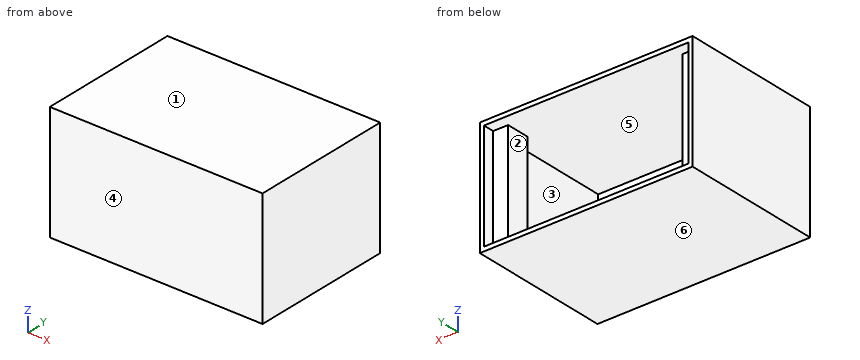
from build123d import *

# Parameters (mm, degrees)
SKETCH1_W           = 456
SKETCH1_H           = 249
SKETCH1_W_2         = 438
SKETCH1_H_2         = 231
BOSS_EXTRUDE1_DEPTH = 9
SKETCH1_3_W         = 456
SKETCH1_3_H         = 249
SKETCH1_3_W_2       = 438
SKETCH1_3_H_2       = 231
BOSS_EXTRUDE2_DEPTH = 298
SKETCH3_W           = 231
SKETCH3_H           = 50
BOSS_EXTRUDE3_DEPTH = 32


with BuildPart() as part:
    # Sketch1 → Boss-Extrude1 (new body)
    with BuildSketch(Plane(origin=(0, 0, 0), x_dir=(1, 0, 0), z_dir=(0, 1, 0))):
        Rectangle(SKETCH1_W, SKETCH1_H)
        Rectangle(SKETCH1_W_2, SKETCH1_H_2, mode=Mode.SUBTRACT)
        Rectangle(SKETCH1_W_2, SKETCH1_H_2)
    extrude(amount=-BOSS_EXTRUDE1_DEPTH)

    # Sketch1<3> → Boss-Extrude2 (add)
    with BuildSketch(Plane(origin=(0, 0, 0), x_dir=(1, 0, 0), z_dir=(0, 1, 0))):
        Rectangle(SKETCH1_3_W, SKETCH1_3_H)
        Rectangle(SKETCH1_3_W_2, SKETCH1_3_H_2, mode=Mode.SUBTRACT)
    extrude(amount=BOSS_EXTRUDE2_DEPTH)

    # Sketch3 → Boss-Extrude3 (add)
    with BuildSketch(Plane(origin=(-219, 0, 0), x_dir=(0, 0, -1), z_dir=(1, 0, 0))):
        with Locations((0, 249)):
            Rectangle(SKETCH3_W, SKETCH3_H)
    boss_extrude3 = extrude(amount=BOSS_EXTRUDE3_DEPTH)

    # Mirror1: Boss-Extrude3 across plane
    add(boss_extrude3.mirror(Plane(origin=(0, 0, 0), x_dir=(0, 0, 1), z_dir=(1, 0, 0))))


solid = part.part
CAD build for the part. Positions are in the model's coordinates, mm. Face numbers are marked on the shaded views. A direction names the side the tool comes from. Give positions to 0.01 mm unless a question says otherwise; leave off trailing zeros. Write each loop counter-clockwise with the first axis right and the second up, starting at its lowest first coordinate (ties: lowest second). Pieces come first, ordered by that corner, then holes. Notation, with made-up numbers: (40, -38) -> (51, -38) arc R11 cw to (51, -23) -> close; hole circle Ø5 at (70, 34.5). An arc over 180 degrees is marked (long way). Return JSON: item names as keys, results as strings.
Item 1: Two-plate mould, pull along Z, no slides. Class the marked faces 3, 4, 5 and 6: +Z half, -Z half, draft (parallel to the pull), parting line (faces both ways), or undercut.
Answer below:
{"face 3": "undercut", "face 4": "draft", "face 5": "undercut", "face 6": "-Z half"}
Item 2: Band-saw the part on C-C (z = 28). List the corners of the cut face in (x, y).
Answer below:
{"outline": "(-228, -9) -> (228, -9) -> (228, 298) -> (219, 298) -> (219, 274) -> (187, 274) -> (187, 224) -> (219, 224) -> (219, 0) -> (-219, 0) -> (-219, 224) -> (-187, 224) -> (-187, 274) -> (-219, 274) -> (-219, 298) -> (-228, 298) -> close"}
Item 3: Band-saw the part on A-A (y = 198.5). List the corners of the cut face in (x, z).
Answer below:
{"outline": "(-228, -124.5) -> (228, -124.5) -> (228, 124.5) -> (-228, 124.5) -> close; hole (-219, -115.5) -> (219, -115.5) -> (219, 115.5) -> (-219, 115.5) -> close"}
Item 4: Drill centre lines: probe 1 along Z at (x, y) = (-37, 21); probe 2 along X at (y, z) = (224.5, -98); probe 3 along X at (y, z) = (161.5, -94.5). Where is each one in solid material? Low to high.
Answer below:
{"probe 1": "z = -124.5 to -115.5, 115.5 to 124.5", "probe 2": "x = -228 to -187, 187 to 228", "probe 3": "x = -228 to -219, 219 to 228"}
Item 5: Drop a flat-ended pin along its axis: pin 1 (16 mm diameter, centred on x = 201.5, z = 57.5, fed in from +Y). Give the stop position or say it passes through.
Answer below:
{"pin 1": "stops at y = 274"}
Item 6: Band-saw the part on B-B (x = 153). List the corners of the cut face in (y, z), then the cut area to 4 significant figures.
Answer below:
{"outline": "(-9, -124.5) -> (298, -124.5) -> (298, -115.5) -> (0, -115.5) -> (0, 115.5) -> (298, 115.5) -> (298, 124.5) -> (-9, 124.5) -> close", "area": "7,605 mm2"}
Item 7: Tool access for the marked faces 1 and 2: list every direction of +Z, -Z, +X, -X, +Y, -Y with a clear straight run to the whole face (end or side of a thin tool).
Answer below:
{"face 1": "+Z, +X, -X, +Y, -Y", "face 2": "+Y"}
